The model under review builds one solid part; all positions refer to its coordinate system, in mm. Face numbers are marked on the shaded views. A direction names the side the tool comes from. Coordinates: 2 decimals unless noted, no trailing zeros. Loops run counter-clockwise (first coordinate to the right, second up) from the corner with the lowest first, then second, coordinate; pieces in that order, holes last. Notation, with made-up numbers: M 22.5,85 L 58.5,85 A33 cw 58.5,115 Z; hole C 80.5,41 d1. An arc over 180 degrees is marked long. One line per item, written item: value.
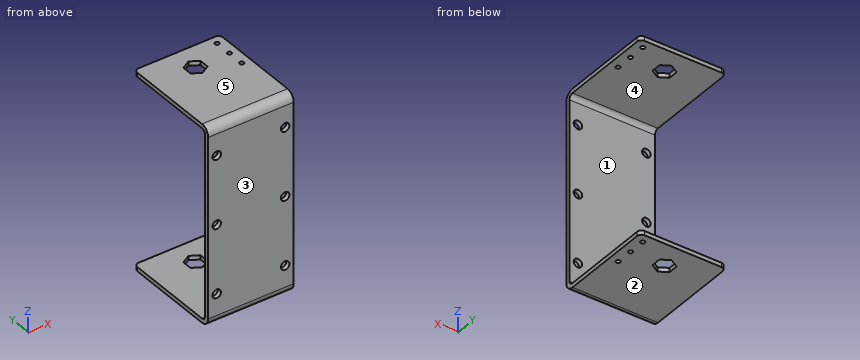
Autodesk Inventor part; units mm, degrees
ref_plane "YZ Plane" through (0, 0, 0) normal (1, 0, 0) x (0, 1, 0)
ref_plane "XZ Plane" through (0, 0, 0) normal (0, 1, 0) x (-1, 0, 0)
ref_plane "XY Plane" through (0, 0, 0) normal (0, 0, 1) x (1, 0, 0)
sketch "Sketch1" plane through (0, 0, 0) normal (0, 0, 1) x (1, 0, 0)
  line L0 (31.75, -38.1) -> (-31.75, -38.1)
  line L1 (-31.75, -38.1) -> (-31.75, 34.925)
  line L2 (-28.575, 38.1) -> (28.575, 38.1)
  line L3 (31.75, 34.925) -> (31.75, -38.1)
  line L4 (31.75, -38.1) -> (-31.75, 38.1) construction
  line L5 (-31.75, -38.1) -> (31.75, 38.1) construction
  arc A0 (31.75, 34.925) -> (28.575, 38.1) centre (28.575, 34.925) ccw
  arc A1 (-28.575, 38.1) -> (-31.75, 34.925) centre (-28.575, 34.925) ccw
  point P0 (0, 0)
  dimension "d0" = 63.5
  dimension "d1" = 76.2
  dimension "d18" = 3.175
extrude "Plate1" add sketch "Sketch1" along normal blind 3.175
sketch "Sketch2" plane through (31.75, -34.925, 0) normal (0, -1, 0) x (1, 0, 0)
  line L0 (-63.5, 0) -> (0, 0)
  line L1 (0, 0) -> (0, 146.05)
  line L2 (0, 146.05) -> (-63.5, 146.05)
  line L3 (-63.5, 146.05) -> (-63.5, 0)
edge flange "Flange1" height 146.05 angle 90 thickness 3.175 bend radius 3.175 thickness toward (0, -1, 0) relief tear relief width 3.175 relief depth 1.5875 edges at (0, -38.1, 3.175) wall of the first edge with corners at (-31.75, -34.925, 0) (31.75, -34.925, 0) (31.75, -34.925, 146.05) (-31.75, -34.925, 146.05)
bend "Bend1"
corner "Corner1"
sketch "Sketch3" plane through (-31.75, -34.925, 146.05) normal (0, 1, 0) x (1, 0, 0)
  circle A0 centre (6.35, 22.225) radius 3.175
  line L0 (0, 0) -> (63.5, 0)
  line L1 (0, 0) -> (0, 139.7)
  line L2 (0, 0) -> (63.5, 0)
  circle A1 centre (6.35, 73.025) radius 3.175
  circle A2 centre (6.35, 123.825) radius 3.175
  circle A3 centre (57.15, 22.225) radius 3.175
  circle A4 centre (57.15, 73.025) radius 3.175
  circle A5 centre (57.15, 123.825) radius 3.175
  point P0 (31.75, 146.05)
  dimension "d13" = 6.35
  dimension "d15" = 6.35
  dimension "d39" = 50.8
  dimension "d42" = 50.8
  dimension "d46" = 22.225
extrude "Cut1" cut sketch "Sketch3" against normal blind 3.175
sketch "Sketch4" plane through (0, 0, 3.175) normal (0, 0, 1) x (1, 0, 0)
  line L0 (-28.575, 38.1) -> (28.575, 38.1)
sketch "Sketch5" plane through (-31.75, -38.1, 146.05) normal (0, 0, 1) x (1, 0, 0)
  line L0 (0, 6.35) -> (0, 73.025)
  arc A0 (3.175, 76.2) -> (0, 73.025) centre (3.175, 73.025) ccw
  line L1 (3.175, 76.2) -> (60.325, 76.2)
  arc A1 (63.5, 73.025) -> (60.325, 76.2) centre (60.325, 73.025) ccw
  line L2 (63.5, 73.025) -> (63.5, 6.35)
  line L3 (0, 0) -> (63.5, 0)
  line L4 (0, 3.175) -> (0, 0)
  line L5 (63.5, 3.175) -> (63.5, 0)
  line L6 (63.5, 3.175) -> (63.5, 6.35)
  line L7 (0, 3.175) -> (0, 6.35)
  line L8 (31.75, 64.4823) -> (38.1, 60.8162)
  line L9 (38.1, 60.8162) -> (38.1, 53.4838)
  line L10 (38.1, 53.4838) -> (31.75, 49.8177)
  line L11 (31.75, 49.8177) -> (25.4, 53.4838)
  line L12 (25.4, 53.4838) -> (25.4, 60.8162)
  line L13 (25.4, 60.8162) -> (31.75, 64.4823)
  point P0 (31.75, 57.15)
  dimension "d51" = 12.7
  dimension "d52" = 19.05
sketch "Sketch6" plane through (31.75, -38.1, 142.875) normal (0, 0, 1) x (1, 0, 0)
  line L0 (-63.5, 0) -> (0, 0)
  line L1 (0, 0) -> (0, 76.2)
  line L2 (0, 76.2) -> (-63.5, 76.2)
  line L3 (-63.5, 76.2) -> (-63.5, 0)
edge flange "Flange2" height 76.2 angle 90 thickness 3.175 bend radius 3.175 thickness toward (0, 0, 1) relief tear relief width 3.175 relief depth 1.5875 edges at (0, -34.925, 146.05) wall of the first edge with corners at (-31.75, -38.1, 142.875) (31.75, -38.1, 142.875) (31.75, 38.1, 142.875) (-31.75, 38.1, 142.875)
bend "Bend2"
corner "Corner2"
fillet "Corner Round1" radius 3.175 2 edges at (-31.75, 38.1, 144.4625) (31.75, 38.1, 144.4625)
extrude "Cut5" cut sketch "Sketch5" against normal blind 3.175 contours L8 L9 L10 L11 L12 L13
sketch "Sketch7" plane through (0, 0, 0) normal (0, 0, -1) x (-1, 0, 0)
  line L0 (0, 26.3823) -> (6.35, 22.7162)
  line L1 (-6.35, 22.7162) -> (0, 26.3823)
  line L2 (-6.35, 15.3838) -> (-6.35, 22.7162)
  line L3 (0, 11.7177) -> (-6.35, 15.3838)
  line L4 (6.35, 15.3838) -> (0, 11.7177)
  line L5 (6.35, 22.7162) -> (6.35, 15.3838)
  point P0 (0, 0)
extrude "Cut6" cut sketch "Sketch7" against normal blind 3.175
sketch "Sketch8" plane through (0, 0, 0) normal (0, 0, -1) x (-1, 0, 0)
  circle A0 centre (-25.273, 31.75) radius 1.5875
  circle A1 centre (-25.273, 19.05) radius 1.5875
  circle A2 centre (-25.273, 6.35) radius 1.5875
  line L0 (31.75, -31.75) -> (31.75, 34.925)
  line L1 (28.575, 38.1) -> (-28.575, 38.1)
  line L2 (-31.75, 34.925) -> (-31.75, -31.75)
  point P0 (0, 0)
  dimension "d57" = 3.175
  dimension "d58" = 3.175
  dimension "d59" = 3.175
  dimension "d61" = 6.35
  dimension "d62" = 12.7
  dimension "d63" = 12.7
  dimension "d68" = 6.477
extrude "Cut7" cut sketch "Sketch8" against normal blind 3.175
sketch "Sketch9" plane through (-31.75, -31.75, 146.05) normal (0, 0, 1) x (1, 0, 0)
  circle A0 centre (57.023, 38.1) radius 1.5875
  circle A1 centre (57.023, 50.8) radius 1.5875
  circle A2 centre (57.023, 63.5) radius 1.5875
  circle A3 centre (57.023, 63.5) radius 1.5875
  circle A4 centre (57.023, 50.8) radius 1.5875
  circle A5 centre (57.023, 38.1) radius 1.5875
  point P0 (31.75, 31.75)
extrude "Cut8" cut sketch "Sketch9" against normal blind 3.175
equation "\"d16\" = Thickness"
equation "\"d53\" = Thickness"
equation "\"d55\" = Thickness"
equation "\"d64\" = Thickness"
equation "\"d66\" = Thickness"
equation "\"d3\" = BendReliefWidth"
equation "\"d4\" = BendReliefDepth"
equation "\"d5\" = MinimumRemnant"
equation "\"d6\" = BendRadius"
equation "\"d9\" = BendRadius"
equation "\"d10\" = CornerReliefSize"
equation "\"d11\" = GapSize"
equation "\"d12\" = JacobiRadiusSize"
equation "\"d24\" = BendReliefWidth"
equation "\"d25\" = BendReliefDepth"
equation "\"d26\" = MinimumRemnant"
equation "\"d27\" = BendRadius"
equation "\"d30\" = BendRadius"
equation "\"d31\" = CornerReliefSize"
equation "\"d32\" = GapSize"
equation "\"d33\" = JacobiRadiusSize"
equation "\"BendRadius\" = Thickness"
equation "\"BendReliefWidth\" = Thickness"
equation "\"BendReliefDepth\" = 0.5 * Thickness"
equation "\"CornerReliefSize\" = 4 * Thickness"
equation "\"MinimumRemnant\" = 2 * Thickness"
equation "\"TransitionRadius\" = BendRadius"
equation "\"JacobiRadiusSize\" = BendRadius"
equation "\"GapSize\" = Thickness"
equation "\"d2\" = BendRadius"
properties part number "334_18_0608_arm connection"
(1) Add section B-B on x = -25.4. State the section outline as (y, z) points (3 decimals).
Checks:
outline: M -38.1,6.35 A6.35 ccw -31.75,0 L 38.1,0 L 38.1,3.175 L -31.75,3.175 A3.175 cw -34.925,6.35 L -34.925,19.05 L -38.1,19.05 Z; M -38.1,25.4 L -34.925,25.4 L -34.925,69.85 L -38.1,69.85 Z; M -38.1,76.2 L -34.925,76.2 L -34.925,120.65 L -38.1,120.65 Z; M -38.1,127 L -34.925,127 L -34.925,139.7 A3.175 cw -31.75,142.875 L 38.1,142.875 L 38.1,146.05 L -31.75,146.05 A6.35 ccw -38.1,139.7 Z
(2) To check wall thickness, follow L1, parallel to Z at x = -27, y = 12.5 (3 decimals); L2, parallel to Z at x = 25.4, y = -35.55; L3, parallel to Z at x = -25, y = -35. State the ranges of each line that lie inside material, in increasing order. Write a range as [from, to].
Checks:
L1: [0, 3.175], [142.875, 146.05]
L2: [1.26, 19.05], [25.4, 69.85], [76.2, 120.65], [127, 144.79]
L3: [0.89, 19.08], [25.37, 69.88], [76.17, 120.68], [126.97, 145.16]
(3) Add section C-C on y = -18. State the section outline as (x, z) points (3 decimals).
Checks:
outline: M -31.75,0 L 31.75,0 L 31.75,3.175 L -31.75,3.175 Z; M -31.75,142.875 L 31.75,142.875 L 31.75,146.05 L -31.75,146.05 Z
(4) Add section A-A on y = 19.05. State how many separate pieces and enclosed holes the cut face has, then the cut area to 3 significant figures.
Checks:
separate pieces: 6
enclosed holes: 0
area: 302 mm^2
(5) Tool access review of the marked faces 1 and 2: name each direction out of +Z, -Z, +X, -X, +Y, -Y from which nothing blocks a thin tool from reaching the whole face with its end or side.
Checks:
face 1: +X, -X, +Y
face 2: -Z, +X, -X, +Y, -Y
(6) Draft analysis for pull direction Z (two halves, no side actions). For the marked faces 3, 4 and 5, state which applies: pulls with the +Z half, pulls with the -Z half, needs draft (parallel to the pull), parting line crosses it, or undercut.
Checks:
face 3: needs draft
face 4: undercut
face 5: pulls with the +Z half
(7) Insertion check: pin 1 Ø4 at (x, y) = (25.273, 6.35) entering from +Z; pin 2 Ø7.5 at (x, z) = (25.4, 123.825) entering from +Y (3 decimals). Each pin has a flat end and moves straight along its axis. Give the tip position at first contact, or say it passes through.
Checks:
pin 1: z = 146.05
pin 2: y = -34.925
